```python
from build123d import *

# Parameters (mm, degrees)
SKETCH2_W           = 250
SKETCH2_H           = 115
SKETCH2_W_2         = 30
SKETCH2_H_2         = 5
BOSS_EXTRUDE1_DEPTH = 5


with BuildPart() as part:
    # Sketch2 → Boss-Extrude1 (new body)
    with BuildSketch(Plane.XY):
        Rectangle(SKETCH2_W, SKETCH2_H)
        with Locations((-94.565217391, 50)):
            Rectangle(SKETCH2_W_2, SKETCH2_H_2, mode=Mode.SUBTRACT)
        with Locations((0.434782609, 50)):
            Rectangle(SKETCH2_W_2, SKETCH2_H_2, mode=Mode.SUBTRACT)
        with Locations((95, 50)):
            Rectangle(SKETCH2_W_2, SKETCH2_H_2, mode=Mode.SUBTRACT)
        with Locations((95, 10)):
            Rectangle(SKETCH2_W_2, SKETCH2_H_2, mode=Mode.SUBTRACT)
        with Locations((0, 10)):
            Rectangle(SKETCH2_W_2, SKETCH2_H_2, mode=Mode.SUBTRACT)
        with Locations((-95, 10)):
            Rectangle(SKETCH2_W_2, SKETCH2_H_2, mode=Mode.SUBTRACT)
        with Locations((-95, -45)):
            Rectangle(SKETCH2_W_2, SKETCH2_H_2, mode=Mode.SUBTRACT)
        with Locations((0, -45)):
            Rectangle(SKETCH2_W_2, SKETCH2_H_2, mode=Mode.SUBTRACT)
        with Locations((95, -45)):
            Rectangle(SKETCH2_W_2, SKETCH2_H_2, mode=Mode.SUBTRACT)
    extrude(amount=BOSS_EXTRUDE1_DEPTH)


solid = part.part
```
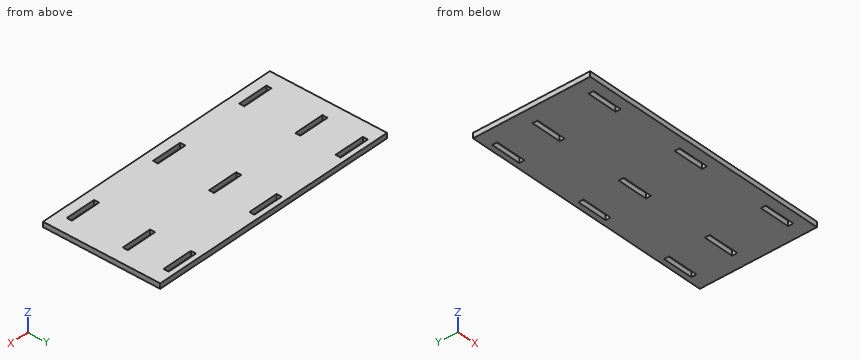
Here's how the part is built. I have some questions about the finished solid (model axes, mm). Give positions to 0.01 mm unless a question says otherwise; leave off trailing zeros. Order: outer loops, then holes, each group sorted by start corner. A loop starts at its lowest first (then second) coordinate and runs counter-clockwise, first axis right, second up. Notation, with made-up numbers: (6, -26) - (20, -26) arc R31 cw to (20, 1) - close; hole circle Ø7 at (89, 42.25). An arc over 180 degrees is marked (long way). Answer as a JSON object with one key per item and string values. Group by question number.
Item 1: If we section it at A-A on x = 5: Please give me the cut outline in (y, z), and give its area (3 significant figures).
Item 2: Please list where these lines run through material, in increasing order: probe 1 along Y at (x, z) = (105, 1.6); probe 2 along X at (y, z) = (8.5, 2.35).
Item 3: If we section it at B-B on z = 3.75: Give the number of separate pieces and of enclosed holes in the cut face, and give its area (3 significant figures).
Result set:
{
 "1": {"outline": "(-57.5, 0) - (-47.5, 0) - (-47.5, 5) - (-57.5, 5) - close; (-42.5, 0) - (7.5, 0) - (7.5, 5) - (-42.5, 5) - close; (12.5, 0) - (47.5, 0) - (47.5, 5) - (12.5, 5) - close; (52.5, 0) - (57.5, 0) - (57.5, 5) - (52.5, 5) - close", "area": "500 mm²"},
 "2": {"probe 1": "-57.5 to -47.5, -42.5 to 7.5, 12.5 to 47.5, 52.5 to 57.5", "probe 2": "-125 to -110, -80 to -15, 15 to 80, 110 to 125"},
 "3": {"separate pieces": "1", "enclosed holes": "9", "area": "27,400 mm²"}
}
